Check sheet for the modelled part. Datum: model origin and axes. Units: mm. Face numbers are marked on the shaded views. A direction names the side the tool comes from. Give positions to 0.01 mm unless a question says otherwise; leave off trailing zeros. Order: outer loops, then holes, each group sorted by start corner. A loop starts at its lowest first (then second) coordinate and runs counter-clockwise, first axis right, second up.
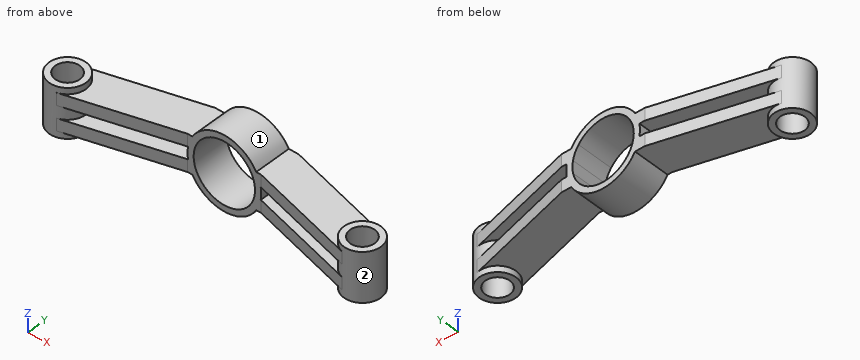
```python
from build123d import *
from build123d.topology import SkipClean

# Parameters (mm, degrees)
SKETCH1_R           = 15
SKETCH1_R_2         = 10
BOSS_EXTRUDE1_DEPTH = 40
BOSS_EXTRUDE2_START = -5
BOSS_EXTRUDE2_DEPTH = 10
BOSS_EXTRUDE3_START = -25
BOSS_EXTRUDE3_DEPTH = 10
SKETCH4_R           = 30
SKETCH4_R_2         = 25
BOSS_EXTRUDE4_DEPTH = 30
CUT_EXTRUDE3_START  = 50
SKETCH5_R           = 25
CUT_EXTRUDE3_DEPTH  = 50


with BuildPart() as part:
    # Sketch1 → Boss-Extrude1 (new body)
    with BuildSketch(Plane.XY):
        with Locations((-120, 0)):
            Circle(SKETCH1_R)
        with Locations((-120, 0)):
            Circle(SKETCH1_R_2, mode=Mode.SUBTRACT)
    extrude(amount=-BOSS_EXTRUDE1_DEPTH)

    # Sketch2 → Boss-Extrude2 (add)
    with BuildSketch(Plane.XY.offset(BOSS_EXTRUDE2_START)):
        with BuildLine():
            Line((0, 38.586284613), (0, 8.586284613))
            Line((0, 8.586284613), (-30, 8.586284613))
            Line((-30, 8.586284613), (-116.117714323, -14.488887394))
            ThreePointArc((-116.117714323, -14.488887394), (-105.511112606, 3.882285677), (-123.882285677, 14.488887394))
            Line((-123.882285677, 14.488887394), (-33.949574928, 38.586284613))
            Line((-33.949574928, 38.586284613), (0, 38.586284613))
        make_face()
    extrude(amount=-BOSS_EXTRUDE2_DEPTH)

    # Sketch3 → Boss-Extrude3 (add)
    with BuildSketch(Plane.XY.offset(BOSS_EXTRUDE3_START)):
        with BuildLine():
            Line((-116.117714323, -14.488887394), (-30, 8.586284613))
            Line((-30, 8.586284613), (0, 8.586284613))
            Line((0, 8.586284613), (0, 38.586284613))
            Line((0, 38.586284613), (-33.949574928, 38.586284613))
            Line((-33.949574928, 38.586284613), (-123.882285677, 14.488887394))
            ThreePointArc((-123.882285677, 14.488887394), (-105.511112606, 3.882285677), (-116.117714323, -14.488887394))
        make_face()
    extrude(amount=-BOSS_EXTRUDE3_DEPTH)

    # Mirror1: part across plane


with BuildPart() as part_1:
    add(part.part)
    add(part.part.mirror(Plane(origin=(0, 0, 0), x_dir=(0, 0, 1), z_dir=(1, 0, 0))))

    # Sketch4 → Boss-Extrude4 (add)
    with BuildSketch(Plane(origin=(0, 38.586284613, 0), x_dir=(1, 0, 0), z_dir=(0, 1, 0))):
        with Locations((0, 20)):
            Circle(SKETCH4_R)
        with Locations((0, 20)):
            Circle(SKETCH4_R_2, mode=Mode.SUBTRACT)
    extrude(amount=-BOSS_EXTRUDE4_DEPTH)

    # Sketch5 → Cut-Extrude3 (cut)
    with SkipClean():  # the faces are left unmerged after this step: merging them gives an invalid solid
        with BuildSketch(Plane(origin=(0, 0, 0), x_dir=(1, 0, 0), z_dir=(0, 1, 0)).offset(CUT_EXTRUDE3_START)):
            with Locations(Location((0, 20, 0), (0, 0, 270))):
                Circle(SKETCH5_R)
        extrude(amount=-CUT_EXTRUDE3_DEPTH, mode=Mode.SUBTRACT)
    add(part_1.part.scale(1), mode=Mode.REPLACE)  # the faces are merged on a copy


solid = part_1.part
```
(1) Set-up check for the marked faces 1 and 2: record each of +Z, -Z, +X, -X, +Y, -Y from which the full face is reachable in a straight line by a thin tool's end or side.
Response values:
face 1: +Z, +Y, -Y
face 2: none
(2) Cross-section at D-D on y = 19. Enter the section's corners in (x, z), then the cut area to 3 significant figures.
Response values:
outline: (-107.05, -35) - (-25.98, -35) arc R30 ccw to (25.98, -35) - (107.05, -35) - (107.05, -25) - (29.58, -25) arc R30 ccw to (29.58, -15) - (107.05, -15) - (107.05, -5) - (25.98, -5) arc R30 ccw to (-25.98, -5) - (-107.05, -5) - (-107.05, -15) - (-29.58, -15) arc R30 ccw to (-29.58, -25) - (-107.05, -25) - close; hole circle Ø50 at (0, -20)
area: 4,020 mm2
(3) Cross-section at B-B on x = 0. Enter the section's corners in (y, z), then the cut area to 3 significant figures.
Response values:
outline: (8.59, -50) - (38.59, -50) - (38.59, -45) - (8.59, -45) - close; (8.59, 5) - (38.59, 5) - (38.59, 10) - (8.59, 10) - close
area: 300 mm2
(4) Material ranges on L1, parallel to Y at x = -120, z = -24; L2, parallel to X at y = 13, z = -4.5; L3, parallel to Z at x = -33, y = 29, recorded low to high.
Response values:
L1: y = -15 to -10, 10 to 15
L2: x = -127.48 to -112.52, -25.69 to -19.62, 19.62 to 25.69, 112.52 to 127.48
L3: z = -35 to -25, -15 to -5
(5) Cross-section at C-C on y = -3. Count the separate pieces of the cut face and the enclosed holes in it, then the cut area to 3 significant figures.
Response values:
separate pieces: 4
enclosed holes: 0
area: 2,110 mm2
(6) Cross-section at A-A on z = -20. Enter the section's corners in (x, y), then the cut area to 3 significant figures.
Response values:
outline: circle Ø30 at (-120, 0); (-30, 8.59) - (-25, 8.59) - (-25, 38.59) - (-30, 38.59) - close; (25, 8.59) - (30, 8.59) - (30, 38.59) - (25, 38.59) - close; circle Ø30 at (120, 0); hole circle Ø20 at (-120, 0); hole circle Ø20 at (120, 0)
area: 1,090 mm2
(7) Gauge pin test, flat ends, axial feed: pin 1 Ø24 at (x, y) = (-119, -1) entering from -Z; pin 2 Ø3 at (x, y) = (57.5, 22.5) entering from +Z; pin 3 Ø1 at (x, y) = (-53.5, 20.5) entering from -Z; pin 4 Ø16 at (x, y) = (120, 0) entering from -Z. Record the tip position at first contact, or that the pin passes through.
Response values:
pin 1: stops at z = -40
pin 2: stops at z = -5
pin 3: stops at z = -35
pin 4: passes through
